CAD build for the part. Positions are in the model's coordinates, mm. A direction names the side the tool comes from. Give positions to 0.01 mm unless a question says otherwise; leave off trailing zeros. Order: outer loops, then holes, each group sorted by start corner. A loop starts at its lowest first (then second) coordinate and runs counter-clockwise, first axis right, second up. Notation, with made-up numbers: M 4,-8 L 40,-8 A4 ccw 40,-2 Z; hole C -7,71 d10. An arc over 180 degrees is marked long. Put each result on its own line as item: value. Start each with the question number.
1) Pin check, flat tips, straight feed: pin 1 (1.5 mm diameter, centred on x = 110, y = -112.5, fed in from +Z); pin 2 (4 mm diameter, centred on x = -140, y = -78.5, fed in from -Z); pin 3 (22.5 mm diameter, centred on y = 68.5, z = 117, fed in from -X). Stop position of each tip, or through.
2) Tool access for faces 1 (the face through (0, -2, 128)), 2 (the face through (0, -2, -74)), 3 (the face through (150, 2, 0)), 4 (the face through (-157, -150, 55)): list every direction of +Z, -Z, +X, -X, +Y, -Y with a clear straight run to the whole face (end or side of a thin tool).
3) Cut at B-B (x = 47.5). Write the cut outline in (y, z), and give its area (3 significant figures).
4) Cut at C-C (z = 95.5). Write the cut outline in (x, y), and give its area (3 significant figures).
5) Two-plate mould, pull along Z, no slides. Class faces 5 (the face through (5, -2, 79)), 6 (the face through (150, 2, 5)), 7 (the face through (-152, 2, 0)): released by +Z, released by -Z, zero draft, split by the parting line, or undercut.
6) Cut at A-A (y = 36). Write the cut outline in (x, z), and give its area (3 significant figures).
7) Drill centre lines: line 1 (X direction, y = -20, z = -82.5); line 2 (Z direction, x = -122.5, y = -30.5). Where is each one in solid material? Low to high. Write a range as [from, to].
```python
from build123d import *

# Parameters (mm, degrees)
F0_W     = 600
F0_H     = 300
F1_DEPTH = 5
F2_W     = 300
F2_H     = 300
F3_DEPTH = 5
F6_W     = 300
F6_H     = 300
F7_DEPTH = 100


# Not quite as in the source:
# - the program builds the solid bodies; features that only make, move or delete a surface that nothing else refers to are left out


with BuildPart() as f1:
    # F0 (on Top) → F1 (new body)
    with BuildSketch(Plane.XY):
        Rectangle(F0_W, F0_H)
    extrude(amount=F1_DEPTH)

    # F2 (on Right) → F3 (join)
    with BuildSketch(Plane.YZ):
        Rectangle(F2_W, F2_H)
    extrude(amount=F3_DEPTH)

    # F6 (on face) → F7 (join)
    with BuildSketch(Plane.XY.offset(5)):
        with Locations((-150, 0)):
            Rectangle(F6_W, F6_H)
    extrude(amount=F7_DEPTH)


solid = f1.part
```
Solution:
1. pin 1: z = 5
1. pin 2: z = 0
1. pin 3: x = 0
2. face 1: +Z, -X, +Y, -Y
2. face 2: -Z, -X, +Y, -Y
2. face 3: -Z, +X, +Y, -Y
2. face 4: +Z, -Z, +X, -X, -Y
3. outline: M -150,0 L 150,0 L 150,5 L -150,5 Z
3. area: 1,500 mm²
4. outline: M -300,-150 L 5,-150 L 5,150 L -300,150 Z
4. area: 91,500 mm²
5. face 5: zero draft
5. face 6: released by +Z
5. face 7: released by -Z
6. outline: M -300,0 L 0,0 L 0,-150 L 5,-150 L 5,0 L 300,0 L 300,5 L 5,5 L 5,150 L 0,150 L 0,105 L -300,105 Z
6. area: 34,500 mm²
7. line 1: [0, 5]
7. line 2: [0, 105]
